```python
from build123d import *

# Parameters (mm, degrees)
SKETCH_2_W               = 1.8
SKETCH_2_H               = 0.7
CHAMFER_1_SIZE           = 1
FILLET_1_R               = 0.4
HOLE_WIZARD_1_D          = 3
PATTERN_CIRCULAR_1_COUNT = 4
SKETCH_5_W               = 2.5
SKETCH_5_H               = 10
CHAMFER_2_SIZE           = 0.6


with BuildPart() as part:
    # Эскиз1 → Повернуть1 (revolve)
    with BuildSketch(Plane.XY, mode=Mode.PRIVATE) as revolve_1_sk:
        Polygon((0, 0), (0, 12.5), (-25, 12.5), (-25, 16), (-28, 16), (-28, 0), align=None)
    revolve(revolve_1_sk.sketch.rotate(Axis((0, 0, 0), (1, 0, 0)), 90), axis=Axis((0, 0, 0), (1, 0, 0)))

    # Эскиз2 → Вырез-Повернуть1 (revolve, cut)
    with BuildSketch(Plane.XY, mode=Mode.PRIVATE) as cut_revolve_1_sk:
        with Locations((-3.1, 12.15)):
            Rectangle(SKETCH_2_W, SKETCH_2_H)
    revolve(cut_revolve_1_sk.sketch.rotate(Axis((0, 0, 0), (-1, 0, 0)), 270), axis=Axis((0, 0, 0), (-1, 0, 0)), mode=Mode.SUBTRACT)

    # Фаска1
    chamfer_1_edges = [part.edges().sort_by_distance(p)[0] for p in [
        (0, 0, -12.5),
    ]]
    chamfer(chamfer_1_edges, length=CHAMFER_1_SIZE)

    # Скругление1
    fillet_1_edges = [part.edges().sort_by_distance(p)[0] for p in [
        (-25, 0, -12.5),
    ]]
    fillet(fillet_1_edges, radius=FILLET_1_R)

    # Отверстие1 (through all)
    with Locations(Plane(origin=(0, 0, 0), x_dir=(0, 0, -1), z_dir=(1, 0, 0))):
        with Locations((4.949747468, 4.949747468)):
            hole_wizard_1 = Hole(HOLE_WIZARD_1_D / 2)

    # Круговой массив1: Отверстие1 ×4 about axis
    pattern_circular_1_axis = Axis((0, 0, 0), (1, 0, 0))
    for i in range(1, PATTERN_CIRCULAR_1_COUNT):
        add(hole_wizard_1.rotate(pattern_circular_1_axis, i * 360 / PATTERN_CIRCULAR_1_COUNT), mode=Mode.SUBTRACT)

    # Эскиз5 → Вырез-Повернуть2 (revolve, cut)
    with BuildSketch(Plane.XY, mode=Mode.PRIVATE) as cut_revolve_2_sk:
        with Locations((-1.25, 5)):
            Rectangle(SKETCH_5_W, SKETCH_5_H)
    revolve(cut_revolve_2_sk.sketch.rotate(Axis((0, 0, 0), (-1, 0, 0)), 90), axis=Axis((0, 0, 0), (-1, 0, 0)), mode=Mode.SUBTRACT)

    # Фаска2
    chamfer_2_edges = [part.edges().sort_by_distance(p)[0] for p in [
        (0, 0, 10),
    ]]
    chamfer(chamfer_2_edges, length=CHAMFER_2_SIZE)


solid = part.part
```
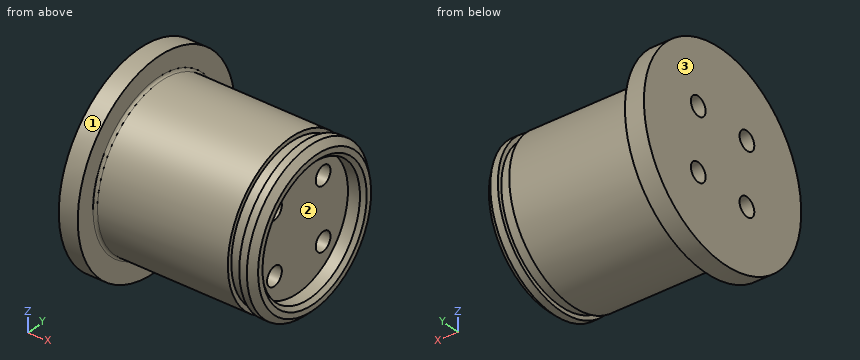
Build history of the part. All positions in model axes, mm. Face numbers are marked on the shaded views. Round coordinates to 2 decimals unless told otherwise and drop trailing zeros. Order: outer loops, then holes, each group sorted by start corner. A loop starts at its lowest first (then second) coordinate and runs counter-clockwise, first axis right, second up. Notation, with made-up numbers: (-25, -26.75) - (14, -26.75) arc R26 cw to (14, 2.25) - close; hole circle Ø2 at (78.5, 71). An arc over 180 degrees is marked (long way). Use a Markdown table: item, result.
1) Saw through at D-D on y = 6. Give the number of separate pieces and of enclosed holes in the cut face, and give its area (3 significant figures).
Recorded:
| item | result |
|---|---|
| separate pieces | 3 |
| enclosed holes | 0 |
| area | 484 mm² |
2) Pull direction Y, two halves, no side cores. Call the marked faces 1, 2 and 3: pulls with the +Y half, pulls with the -Y half, needs draft (parallel to the pull), parting line crosses it, or undercut.
Recorded:
| item | result |
|---|---|
| face 1 | parting line crosses it |
| face 2 | undercut |
| face 3 | needs draft |
3) Saw through at C-C on x = -22.25. Write the cut outline in (y, z).
Recorded:
| item | result |
|---|---|
| outline | circle Ø25 at (0, 0); hole circle Ø3 at (-4.95, -4.95); hole circle Ø3 at (-4.95, 4.95); hole circle Ø3 at (4.95, -4.95); hole circle Ø3 at (4.95, 4.95) |
4) Flat gauge pins, fed straight in: pin 1 Ø3 at (x, z) = (-14.5, 8.5) entering from +Y; pin 2 Ø4 at (y, z) = (-4.95, 4.95) entering from +X; pin 3 Ø1 at (x, y) = (-24, 5) entering from -Z. Where does each tip first touch, or does it go through?
Recorded:
| item | result |
|---|---|
| pin 1 | stops at y = 10.36 |
| pin 2 | stops at x = -2.5 |
| pin 3 | stops at z = -11.66 |
5) Saw through at A-A on y = 0. Write the cut outline in (x, z).
Recorded:
| item | result |
|---|---|
| outline | (-28, -16) - (-25, -16) - (-25, -12.9) arc R0.4 cw to (-24.6, -12.5) - (-4, -12.5) - (-4, -11.8) - (-2.2, -11.8) - (-2.2, -12.5) - (-1, -12.5) - (0, -11.5) - (0, -10.6) - (-0.6, -10) - (-2.5, -10) - (-2.5, 10) - (-0.6, 10) - (0, 10.6) - (0, 11.5) - (-1, 12.5) - (-2.2, 12.5) - (-2.2, 11.8) - (-4, 11.8) - (-4, 12.5) - (-24.6, 12.5) arc R0.4 cw to (-25, 12.9) - (-25, 16) - (-28, 16) - close |
6) Wall check: L1, parallel to Z at x = -14.25, y = -6; L2, parallel to Z at x = -17.5, y = 5.5; L3, parallel to X at y = -7.5, z = -9.5. Give the ranges that are in metal, low to high.
Recorded:
| item | result |
|---|---|
| L1 | z = -10.97 to -6.02, -3.88 to 3.88, 6.02 to 10.97 |
| L2 | z = -11.22 to -6.35, -3.55 to 3.55, 6.35 to 11.22 |
| L3 | x = -28 to -4, -2.2 to -0.6 |
